Answer from the drawing. Dimensions are ordinates in mm from the lowest x, y and z of the part. Round coordinates to 2 decimals unless told otherwise and drop trailing zeros. Write each loop counter-clockwise with the first axis right and the second up, starting at its lowest first coordinate (ties: lowest second). Pieces come first, ordered by that corner, then holes.
1. Find section A-A (x = 431.8). Write down the section's boundary in (y, z).
2. Find section B-B (z = 50.8). Count the separate pieces of the cut face and the enclosed holes in it, and give its area (3 significant figures).
3. Straight lines are drawn through the part: probe 1 along Z at (x, y) = (558.8, 6); probe 2 along Z at (x, y) = (53.5, 5.25). For each, find the intervals that lie inside material, in ascending order.
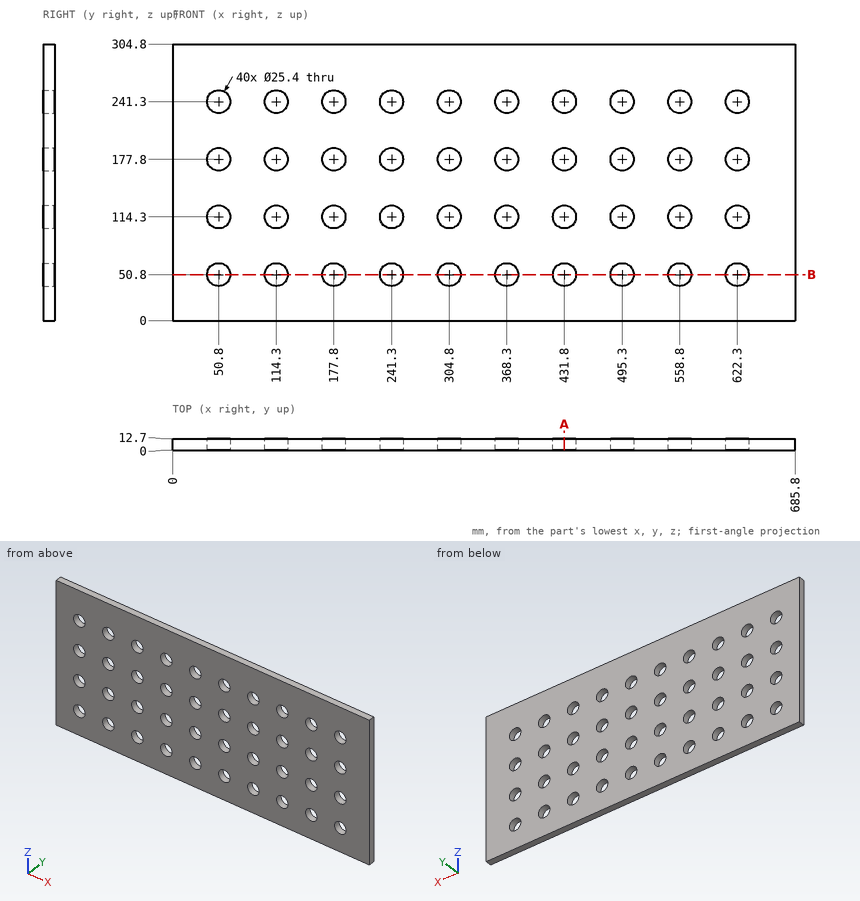
Worked answers:
1. outline: (0, 0) - (12.7, 0) - (12.7, 38.1) - (0, 38.1) - close; (0, 63.5) - (12.7, 63.5) - (12.7, 101.6) - (0, 101.6) - close; (0, 127) - (12.7, 127) - (12.7, 165.1) - (0, 165.1) - close; (0, 190.5) - (12.7, 190.5) - (12.7, 228.6) - (0, 228.6) - close; (0, 254) - (12.7, 254) - (12.7, 304.8) - (0, 304.8) - close
2. separate pieces: 11
2. enclosed holes: 0
2. area: 5,480 mm2
3. probe 1: z = 0 to 38.1, 63.5 to 101.6, 127 to 165.1, 190.5 to 228.6, 254 to 304.8
3. probe 2: z = 0 to 38.39, 63.21 to 101.89, 126.71 to 165.39, 190.21 to 228.89, 253.71 to 304.8
